```python
from build123d import *

# Parameters (mm, degrees)
F_1_4_20_TAPPED_HOLE1_D           = 5.1054
F_1_4_20_TAPPED_HOLE1_CSINK_D     = 7.62
F_1_4_20_TAPPED_HOLE1_CSINK_ANGLE = 100


with BuildPart() as part:
    # Sketch1 → Revolve1 (revolve)
    with BuildSketch(Plane.XY):
        Polygon((0, 0), (0, -19.05), (-25.4, -19.05), (-25.4, -25.4), (-31.75, -25.4), (-31.75, 0), align=None)
    revolve(axis=Axis((-45.965152255, 0, 0), (1, 0, 0)))

    # 1/4-20 Tapped Hole1 (through all)
    with Locations(Plane.ZY.offset(31.75)):
        with Locations((0, 0)):
            CounterSinkHole(F_1_4_20_TAPPED_HOLE1_D / 2, F_1_4_20_TAPPED_HOLE1_CSINK_D / 2, counter_sink_angle=F_1_4_20_TAPPED_HOLE1_CSINK_ANGLE)


solid = part.part
```
Geometry: final body of the model. Coordinates: model frame, mm. A direction names the side the tool comes from. Coordinates: 2 decimals unless noted, no trailing zeros. Order: outer loops, then holes, each group sorted by start corner. A loop starts at its lowest first (then second) coordinate and runs counter-clockwise, first axis right, second up.
Item 1: Section query D-D (x = -16.5). Output: boundary loops of the cut face in (y, z), then the cut area to 3 significant figures.
Answer:
outline: circle Ø38.1 at (0, 0); hole circle Ø5.11 at (0, 0)
area: 1,120 mm2
Item 2: Contact query for flat-ended pins moving along their axis: P1, Ø3, axis at x = -22.5, y = 18, coming from the -Z side; P2, Ø2, axis at x = -10, y = 9, coming from the -Z side; P3, Ø1, axis at x = -4.5, y = 5.5, coming from the -Z side; P4, Ø4.5, axis at y = 0, z = 0, coming from the -X side. Output: stop coordinate, or through.
Answer:
P1: stops at z = -9.52
P2: stops at z = -17.29
P3: stops at z = -18.38
P4: passes through
Item 3: Material intervals for line 1 along Y through (x, z) = (-24, 0); line 2 along Z through (x, y) = (-5, 0.5), sorted ascending.
Answer:
line 1: y = -19.05 to -2.55, 2.55 to 19.05
line 2: z = -19.04 to -2.5, 2.5 to 19.04
Item 4: Section query C-C (z = -8). Output: boundary loops of the cut face in (x, y), then the cut area to 3 significant figures.
Answer:
outline: (-31.75, -24.11) - (-25.4, -24.11) - (-25.4, -17.29) - (0, -17.29) - (0, 17.29) - (-25.4, 17.29) - (-25.4, 24.11) - (-31.75, 24.11) - close
area: 1,180 mm2
Item 5: Section query A-A (z = 0). Output: boundary loops of the cut face in (x, y) (3 decimals).
Answer:
outline: (-31.75, -25.4) - (-25.4, -25.4) - (-25.4, -19.05) - (0, -19.05) - (0, -2.553) - (-30.695, -2.553) - (-31.75, -3.81) - close; (-31.75, 3.81) - (-30.695, 2.553) - (0, 2.553) - (0, 19.05) - (-25.4, 19.05) - (-25.4, 25.4) - (-31.75, 25.4) - close
Item 6: Draft query along Y for faces 1 (the face through (0, 4, 0)), 2 (the face through (-12.88, 15.12, 11.59)), 3 (the face through (-15.133, 0.767, -2.435)). Return one class per face: released by +Y, released by -Y, zero draft, split by the parting line, or undercut.
Answer:
face 1: zero draft
face 2: split by the parting line
face 3: undercut
Item 7: Access query for faces 4 (the face through (-25.4, 4, -19)), 5 (the face through (-31.75, -5, 0)). Directions: +Z, -Z, +X, -X, +Y, -Y. A direction counts if a zero-diameter tool reaches every point of the face in a straight line with its end or side. Return the directions, or none.
Answer:
face 4: +X
face 5: +Z, -Z, -X, +Y, -Y
